Geometry: see drawing. Coordinates: mm, zero at the bounding-box minimum. Coordinates: 2 decimals unless noted, no trailing zeros. Write each loop counter-clockwise with the first axis right and the second up, starting at its lowest first coordinate (ties: lowest second). Pieces come first, ordered by that corner, then holes.
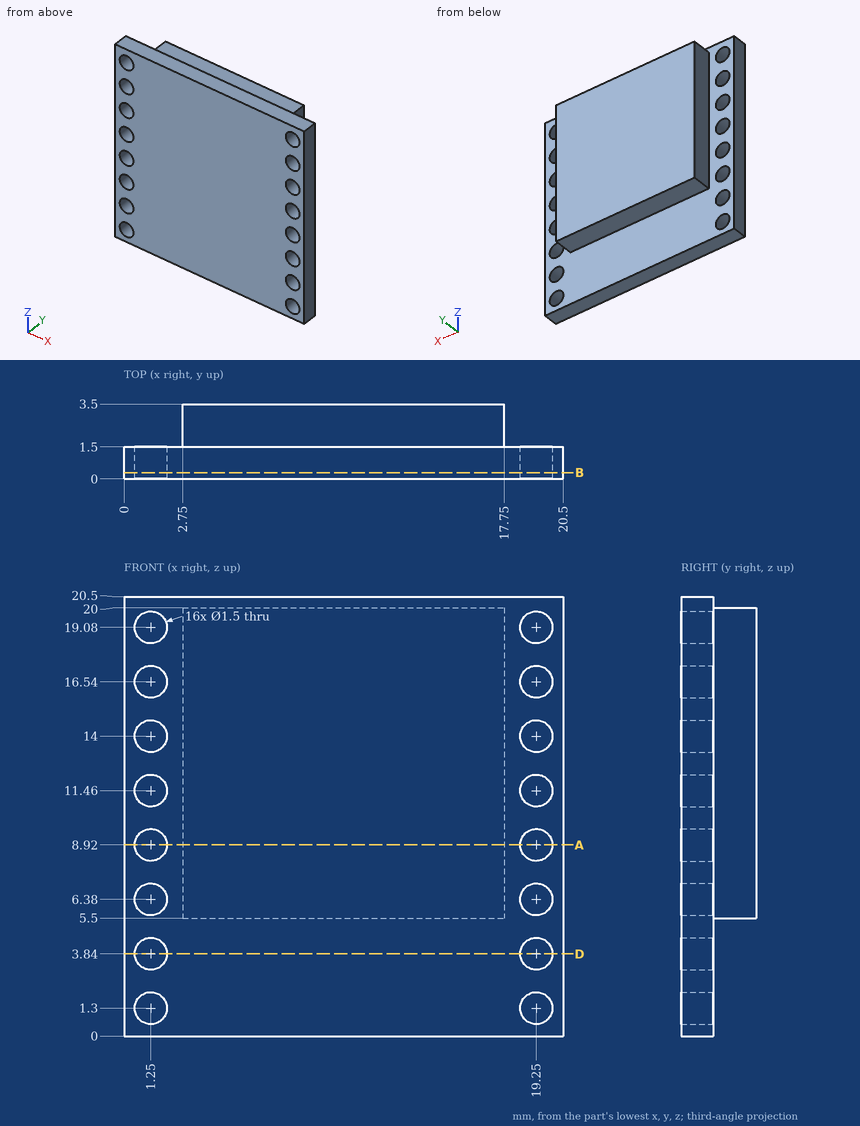
Item 1: Section B-B, the plane y = 0.3. State how many separate pieces and enclosed holes the cut face has, plus the area to 3 significant figures.
Derived:
separate pieces: 1
enclosed holes: 16
area: 392 mm2
Item 2: Section A-A, the plane z = 8.92. Output: boundary loops of the cut face in (x, y).
Derived:
outline: (0, 0) - (0.5, 0) - (0.5, 1.5) - (0, 1.5) - close; (2, 0) - (18.5, 0) - (18.5, 1.5) - (17.75, 1.5) - (17.75, 3.5) - (2.75, 3.5) - (2.75, 1.5) - (2, 1.5) - close; (20, 0) - (20.5, 0) - (20.5, 1.5) - (20, 1.5) - close
Item 3: Section D-D, the plane z = 3.84. Output: boundary loops of the cut face in (x, y), plus the area to 4 significant figures.
Derived:
outline: (0, 0) - (0.5, 0) - (0.5, 1.5) - (0, 1.5) - close; (2, 0) - (18.5, 0) - (18.5, 1.5) - (2, 1.5) - close; (20, 0) - (20.5, 0) - (20.5, 1.5) - (20, 1.5) - close
area: 26.25 mm2
Item 4: Material intervals for probe 1 along X at (y, z) = (0.35, 14); probe 2 along X at (y, z) = (0.7, 3.25); probe 3 along Z at (x, y) = (7, 2.05), sorted ascending.
Derived:
probe 1: x = 0 to 0.5, 2 to 18.5, 20 to 20.5
probe 2: x = 0 to 0.79, 1.71 to 18.79, 19.71 to 20.5
probe 3: z = 5.5 to 20
Item 5: Pin query (flat end, axial travel): pin 1 (2.5 mm diameter, centred on x = 19.25, z = 1.3, fed in from +Y); pin 2 (1 mm diameter, centred on y = 2.5, z = 7, fed in from -X); pin 3 (0.6 mm diameter, centred on x = 13, y = 2, fed in from -Z). Return the tip coordinate at first contact, or that it passes through.
Derived:
pin 1: stops at y = 1.5
pin 2: stops at x = 2.75
pin 3: stops at z = 5.5
